The drawing under review shows one solid part. Ordinate dimensions are in mm from its lowest x, y, z. A direction names the side the tool comes from. Round coordinates to 2 decimals unless told otherwise and drop trailing zeros. Write each loop counter-clockwise with the first axis right and the second up, starting at its lowest first coordinate (ties: lowest second). Pieces come first, ordered by that corner, then holes. Notation, with made-up numbers: (26.5, 81) -> (54.5, 81) arc R37 ccw to (54.5, 120) -> close; hole circle Ø8 at (82.25, -21.75). An arc over 180 degrees is marked (long way). Answer in a Markdown table with one row per item. Add a question column.
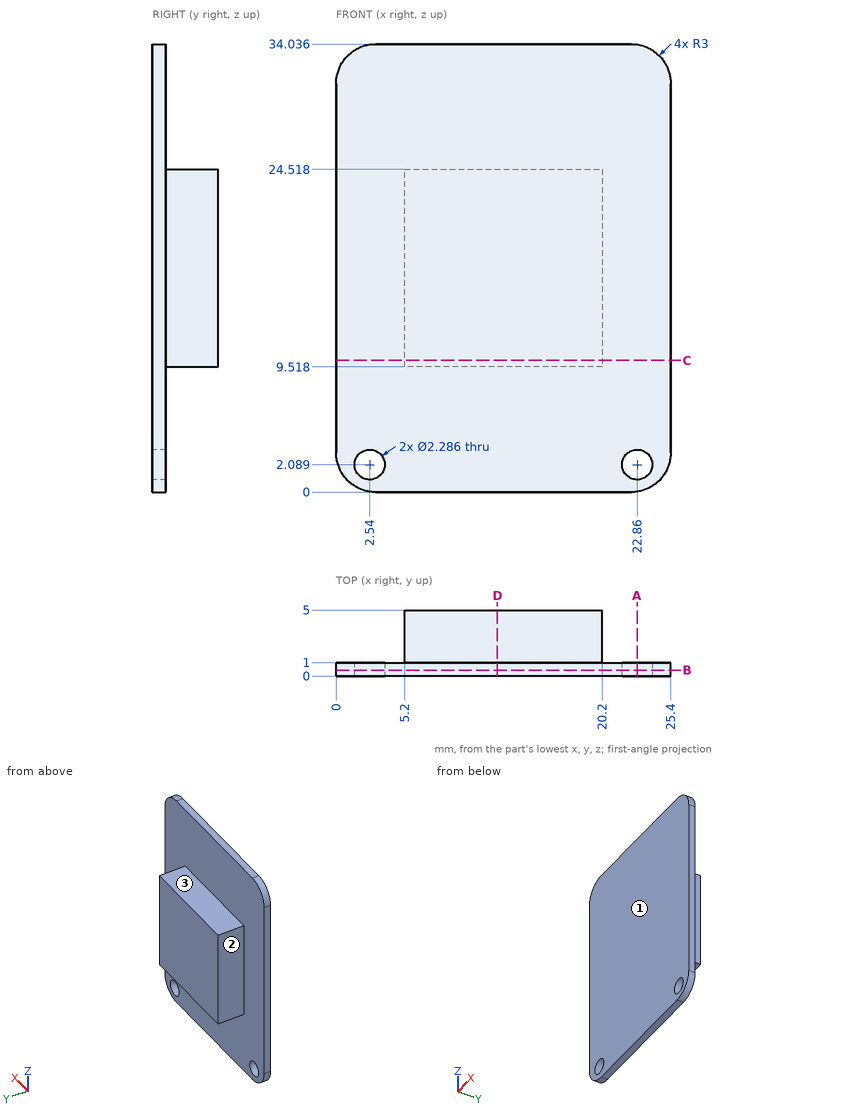
1. For L1, parallel to X at y = 0.5, z = 3; L2, parallel to X at y = 3.65, z = 16.5; L3, parallel to Z at x = 10.5, y = 1.7, list the stretches that pass through material, from the lowest coordinate up.
2. Insertion check: pin 1 Ø4 at (x, z) = (12, 27) entering from +Y; pin 2 Ø1.2 at (y, z) = (2, 18.5) entering from -X; pin 3 Ø2 at (y, z) = (2.5, 14) entering from +X. Each pin has a flat end and moves straight along its axis. Give the tip position at first contact, or say it passes through.
3. Add section A-A on x = 22.86. Write out the cut boundary in (y, z).
4. Tool access review of the marked faces 1, 2 and 3: name each direction out of +Z, -Z, +X, -X, +Y, -Y from which nothing blocks a thin tool from reaching the whole face with its end or side.
5. Add section B-B on y = 0.45. Write out the cut boundary in (x, z), plus the area to 3 significant figures.
6. Add section C-C on z = 10. Write out the cut boundary in (x, y), plus the area to 3 significant figures.
7. Add section D-D on x = 12.25. Write out the cut boundary in (y, z).
Filled in:
| question | item | result |
|---|---|---|
| 1 | L1 | 0 to 1.85, 3.23 to 22.17, 23.55 to 25.4 |
| 1 | L2 | 5.2 to 20.2 |
| 1 | L3 | 9.52 to 24.52 |
| 2 | pin 1 | y = 1 |
| 2 | pin 2 | x = 5.2 |
| 2 | pin 3 | x = 20.2 |
| 3 | outline | (0, 0.04) -> (1, 0.04) -> (1, 0.95) -> (0, 0.95) -> close; (0, 3.23) -> (1, 3.23) -> (1, 34) -> (0, 34) -> close |
| 4 | face 1 | +Z, -Z, +X, -X, -Y |
| 4 | face 2 | +Z, -Z, -X, +Y |
| 4 | face 3 | +Z, +X, -X, +Y |
| 5 | outline | (0, 3) arc R3 ccw to (3, 0) -> (22.4, 0) arc R3 ccw to (25.4, 3) -> (25.4, 31.04) arc R3 ccw to (22.4, 34.04) -> (3, 34.04) arc R3 ccw to (0, 31.04) -> close; hole circle Ø2.29 at (2.54, 2.09); hole circle Ø2.29 at (22.86, 2.09) |
| 5 | area | 849 mm² |
| 6 | outline | (0, 0) -> (25.4, 0) -> (25.4, 1) -> (20.2, 1) -> (20.2, 5) -> (5.2, 5) -> (5.2, 1) -> (0, 1) -> close |
| 6 | area | 85.4 mm² |
| 7 | outline | (0, 0) -> (1, 0) -> (1, 9.52) -> (5, 9.52) -> (5, 24.52) -> (1, 24.52) -> (1, 34.04) -> (0, 34.04) -> close |
